from build123d import *

# Parameters (mm, degrees)
RESSALTO_EXTRUS_O1_DEPTH      = 10
RESSALTO_EXTRUS_O1_DEPTH_BACK = 30
ESBO_O1_R                     = 23.59
RESSALTO_EXTRUS_O2_DEPTH      = 30
CORTE_EXTRUS_O1_DEPTH         = 59.405
CORTE_EXTRUS_O2_DEPTH         = 79.405
SKETCH2_R                     = 2.5
CUT_EXTRUDE1_DEPTH            = 80.519934634


with BuildPart() as part:
    # Esboço1 → Ressalto-extrusão1 (new, two sides: drawn at the far end of the back side and taken through both)
    with BuildSketch(Plane.XY.offset(-RESSALTO_EXTRUS_O1_DEPTH_BACK)):
        Circle(ESBO_O1_R)
    extrude(amount=RESSALTO_EXTRUS_O1_DEPTH + RESSALTO_EXTRUS_O1_DEPTH_BACK)

    # Esboço2 → Ressalto-extrusão2 (add)
    with BuildSketch(Plane(origin=(0, 0, -30), x_dir=(-1, 0, 0), z_dir=(0, 0, -1))):
        Polygon((-7.5, -15.101129972), (-7.5, 0), (-7.5, 15.101129972), (-18.123023301, 15.101129972), (-18.123023301, -15.101129972), align=None)
        Polygon((7.5, -15.101129972), (7.5, 0), (7.5, 15.101129972), (18.123023301, 15.101129972), (18.123023301, -15.101129972), align=None)
    extrude(amount=RESSALTO_EXTRUS_O2_DEPTH)

    # Esboço3 → Corte-extrusão1 (cut, symmetric)
    with BuildSketch(Plane.ZY.offset(18.123023301)):
        with BuildLine():
            Line((-44.405, 18.172432148), (-62.563044424, 18.172432148))
            Line((-62.563044424, 18.172432148), (-62.563044424, -18.251867877))
            Line((-62.563044424, -18.251867877), (-44.405, -18.251867877))
            Line((-44.405, -18.251867877), (-44.405, -15.101129972))
            ThreePointArc((-44.405, -15.101129972), (-59.506129972, 0), (-44.405, 15.101129972))
            Line((-44.405, 15.101129972), (-44.405, 18.172432148))
        make_face()
    extrude(amount=CORTE_EXTRUS_O1_DEPTH, both=True, mode=Mode.SUBTRACT)

    # Esboço4 → Corte-extrusão2 (cut, symmetric)
    with BuildSketch(Plane.ZY.offset(18.123023301)):
        with BuildLine():
            Line((-46.190357107, 1.75), (-42.619642893, 1.75))
            ThreePointArc((-42.619642893, 1.75), (-41.905, 0), (-42.619642893, -1.75))
            Line((-42.619642893, -1.75), (-46.190357107, -1.75))
            ThreePointArc((-46.190357107, -1.75), (-46.905, 0), (-46.190357107, 1.75))
        make_face()
    extrude(amount=CORTE_EXTRUS_O2_DEPTH, both=True, mode=Mode.SUBTRACT)

    # Sketch2 → Cut-Extrude1 (cut, through all)
    with BuildSketch(Plane(origin=(0, 23.59, 0), x_dir=(1, 0, 0), z_dir=(0, 1, 0))):
        with Locations(Location((0, 2.99, 0), (0, 0, 270))):
            Circle(SKETCH2_R)
    extrude(amount=-CUT_EXTRUDE1_DEPTH, mode=Mode.SUBTRACT)


solid = part.part
Check sheet for the modelled part. Datum: model origin and axes. Units: mm. A direction names the side the tool comes from. Give positions to 0.01 mm unless a question says otherwise; leave off trailing zeros. Write each loop counter-clockwise with the first axis right and the second up, starting at its lowest first coordinate (ties: lowest second). Pieces come first, ordered by that corner, then holes. Notation, with made-up numbers: (21, -22) -> (48, -22) arc R21 cw to (48, -10) -> close; hole circle Ø4 at (11.5, 47). An arc over 180 degrees is marked (long way). Write item = value, one per line.
Item 1: Tool access check on faces 1 (the flat face through (13, -15.101, -37)), 2 (the flat face through (7.5, 0, -41)), 3 (the cylindrical face through (-12.886, 0.027, -41.905)), 4 (the flat face through (-20, 0, -30)). Record the directions out of +Z, -Z, +X, -X, +Y, -Y that give a thin tool (end or side, any length) a straight path to the whole face; none if there is none.
Output:
face_1 = -Z, +X, -X, -Y
face_2 = -Z, +Y, -Y
face_3 = +X, -X
face_4 = -Z, -X, +Y, -Y
Item 2: Sectioned sample at D-D on y = 6.5. Record the boundary of the cut face in (x, z).
Output:
outline = (-22.68, -30) -> (-18.12, -30) -> (-18.12, -58.04) -> (-7.5, -58.04) -> (-7.5, -30) -> (7.5, -30) -> (7.5, -58.04) -> (18.12, -58.04) -> (18.12, -30) -> (22.68, -30) -> (22.68, 10) -> (-22.68, 10) -> close; hole circle Ø5 at (0, -2.99)
Item 3: Gauge pin test, flat ends, axial feed: pin 1 (8.5 mm diameter, centred on x = -13, z = -37, fed in from -Y); pin 2 (11.5 mm diameter, centred on x = -10, z = -37.5, fed in from +Y); pin 3 (3 mm diameter, centred on y = 15, z = -9, fed in from -X). Record the tip position at first contact, or that the pin passes through.
Output:
pin_1 = -15.1
pin_2 = 15.1
pin_3 = -19.35
Item 4: Scan lines: probe 1 along X at (y, z) = (-2, -51); probe 2 along X at (y, z) = (0, -2.99); probe 3 along Z at (x, y) = (0, -9.5). Record each from-to range of solid material in increasing order. Write a range as from..to.
Output:
probe_1 = -18.12..-7.5, 7.5..18.12
probe_2 = -23.59..-2.5, 2.5..23.59
probe_3 = -30..-5.49, -0.49..10
Item 5: Sectioned sample at B-B on x = 0. Record the boundary of the cut face in (y, z).
Output:
outline = (-23.59, -30) -> (23.59, -30) -> (23.59, -5.49) -> (-23.59, -5.49) -> close; (-23.59, -0.49) -> (23.59, -0.49) -> (23.59, 10) -> (-23.59, 10) -> close
Item 6: Release check for a two-part mould opening along Y. For faces 5 (the cylindrical face through (12.737, 0.027, -41.905)), 6 (the flat face through (13, 15.101, -37)), 7 (the flat face through (20, 0, -30)), 8 (the flat face through (13, -1.75, -44)) record: +Y half, -Y half, draft (parallel to the pull), parting line (faces both ways), or undercut.
Output:
face_5 = undercut
face_6 = +Y half
face_7 = draft
face_8 = undercut
Item 7: Sectioned sample at A-A on y = 0. Record the boundary of the cut face in (x, z) (3 decimals).
Output:
outline = (-23.59, -30) -> (-18.123, -30) -> (-18.123, -41.905) -> (-7.5, -41.905) -> (-7.5, -30) -> (7.5, -30) -> (7.5, -41.905) -> (18.123, -41.905) -> (18.123, -30) -> (23.59, -30) -> (23.59, 10) -> (-23.59, 10) -> close; (-18.123, -59.506) -> (-7.5, -59.506) -> (-7.5, -46.905) -> (-18.123, -46.905) -> close; (7.5, -59.506) -> (18.123, -59.506) -> (18.123, -46.905) -> (7.5, -46.905) -> close; hole circle Ø5 at (0, -2.99)
Item 8: Sectioned sample at C-C on z = -35.5. Record the boundary of the cut face in (x, y).
Output:
outline = (-18.12, -15.1) -> (-7.5, -15.1) -> (-7.5, 15.1) -> (-18.12, 15.1) -> close; (7.5, -15.1) -> (18.12, -15.1) -> (18.12, 15.1) -> (7.5, 15.1) -> close
